Model file for the job. Use its own axes, mm. A direction names the side the tool comes from. Coordinates: 2 decimals unless noted, no trailing zeros. Write each loop counter-clockwise with the first axis right and the second up, starting at its lowest first coordinate (ties: lowest second). Pieces come first, ordered by that corner, then holes. Notation, with made-up numbers: M -39.75,11 L 15.25,11 A20 cw 15.25,41 Z; hole C 53.25,65.25 d1. An arc over 180 degrees is marked long. Answer in a Markdown table with one row per item. Add a question column.
```python
from build123d import *

# Parameters (mm, degrees)
F3_DEPTH = 6.6
F4_SIZE  = 0.5


with BuildPart() as f1:
    # F0 (on Front) → F1 (revolve)
    with BuildSketch(Plane.XZ):
        Polygon((8.457855, 12), (0, 12), (0, -30), (6, -30), (6, 0), (8.411715, 0), (9, 0.542145), (9, 11.411715), align=None)
    revolve(axis=Axis((0, 0, -9), (0, 0, 1)))

    # F2 (on face) → F3 (cut)
    with BuildSketch(Plane.XY.offset(12)):
        Polygon((-1.227341, 5.641539), (-5.499387, 1.757861), (-4.272046, -3.883678), (1.227341, -5.641539), (5.499387, -1.757861), (4.272046, 3.883678), align=None)
    extrude(amount=-F3_DEPTH, mode=Mode.SUBTRACT)

    # F4
    f4_edges = [f1.edges().sort_by_distance(p)[0] for p in [
        (3.363364, -3.6997, 12),
        (-1.522352, -4.762609, 12),
        (-4.885716, -1.062909, 12),
        (-3.363364, 3.6997, 12),
        (1.522352, 4.762609, 12),
        (4.885716, 1.062909, 12),
        (4.885716, 1.062909, 5.4),
        (3.363364, -3.6997, 5.4),
        (-1.522352, -4.762609, 5.4),
        (-4.885716, -1.062909, 5.4),
        (-3.363364, 3.6997, 5.4),
        (1.522352, 4.762609, 5.4),
    ]]
    chamfer(f4_edges, length=F4_SIZE)


solid = f1.part
```
1) Slice it at B-B (y = 0). Give the cut face in (x, z), then the cut area to 3 significant figures.
2) Which spindle directions (+Z, -Z, +X, -X, +Y, -Y) get a long thin tool onto all of the face, cutting with end or side? Do faces 1 (the face through (0, 0, -30)), 2 (the face through (-1.64, -4.984, 11.746)). Say none if no direction does.
3) Drill centre lines: probe 1 along Z at (x, y) = (3.5, -2.25); probe 2 along Z at (x, y) = (6.75, -0.75); probe 3 along X at (y, z) = (-0.25, -19.5). Where is each one in solid material? Low to high.
4) Slice it at D-D (z = -13.5). Give the cut face in (x, y).
5) Flat gauge pins, fed straight in: pin 1 Ø4 at (x, z) = (6.5, -1) entering from -Y; pin 2 Ø10 at (y, z) = (5, -22.5) entering from +X; pin 3 Ø1 at (x, z) = (5.5, -12) entering from -Y. Where does each tip first touch, or does it go through?
6) Slice it at C-C (x = 0). Give the cut face in (y, z), then the cut area to 3 significant figures.
7) Two-plate mould, pull along X, no slides. Class faces 3 (the face through (-2, -6, 12)), 4 (the face through (-3.33, 3.73, 8.74)), 5 (the face through (-1.172, 8.923, 6.053)): released by +X, released by -X, zero draft, split by the parting line, or undercut.
8) Slice it at A-A (z = 8.5). Give the cut face in (x, y), then the cut area to 3 significant figures.
Ans:
| question | item | result |
|---|---|---|
| 1 | outline | M -9,0.54 L -8.41,0 L -6,0 L -6,-30 L 6,-30 L 6,0 L 8.41,0 L 9,0.54 L 9,11.41 L 8.46,12 L 5.63,12 L 5.12,11.5 L 5.12,5.9 L 4.61,5.4 L -4.61,5.4 L -5.12,5.9 L -5.12,11.5 L -5.63,12 L -8.46,12 L -9,11.41 Z |
| 1 | area | 508 mm2 |
| 2 | face 1 | -Z, +X, -X, +Y, -Y |
| 2 | face 2 | +Z |
| 3 | probe 1 | z = -30 to 5.4 |
| 3 | probe 2 | z = 0 to 12 |
| 3 | probe 3 | x = -5.99 to 5.99 |
| 4 | outline | C 0,0 d12 |
| 5 | pin 1 | stops at y = -7.33 |
| 5 | pin 2 | stops at x = 6 |
| 5 | pin 3 | stops at y = -3.32 |
| 6 | outline | M -9,0.54 L -8.41,0 L -6,0 L -6,-30 L 6,-30 L 6,0 L 8.41,0 L 9,0.54 L 9,11.41 L 8.46,12 L 5.77,12 L 5.25,11.5 L 5.25,5.9 L 4.72,5.4 L -4.72,5.4 L -5.25,5.9 L -5.25,11.5 L -5.77,12 L -8.46,12 L -9,11.41 Z |
| 6 | area | 506 mm2 |
| 7 | face 3 | zero draft |
| 7 | face 4 | undercut |
| 7 | face 5 | split by the parting line |
| 8 | outline | C 0,0 d18; hole M -5.5,1.76 L -4.27,-3.88 L 1.23,-5.64 L 5.5,-1.76 L 4.27,3.88 L -1.23,5.64 Z |
| 8 | area | 168 mm2 |
